Here's the drawing with two shaded views (mm, measured from the low corner). I have some questions. Coordinates: 2 decimals unless noted, no trailing zeros. Write each loop counter-clockwise with the first axis right and the second up, starting at its lowest first coordinate (ties: lowest second). Pieces come first, ordered by that corner, then holes. Notation, with made-up numbers: (78.25, -22) -> (85.25, -22) arc R18 cw to (85.25, 7) -> close; hole circle Ø6 at (-23, 7.25). An arc over 180 degrees is marked (long way). Put each result on its own line as item: value.
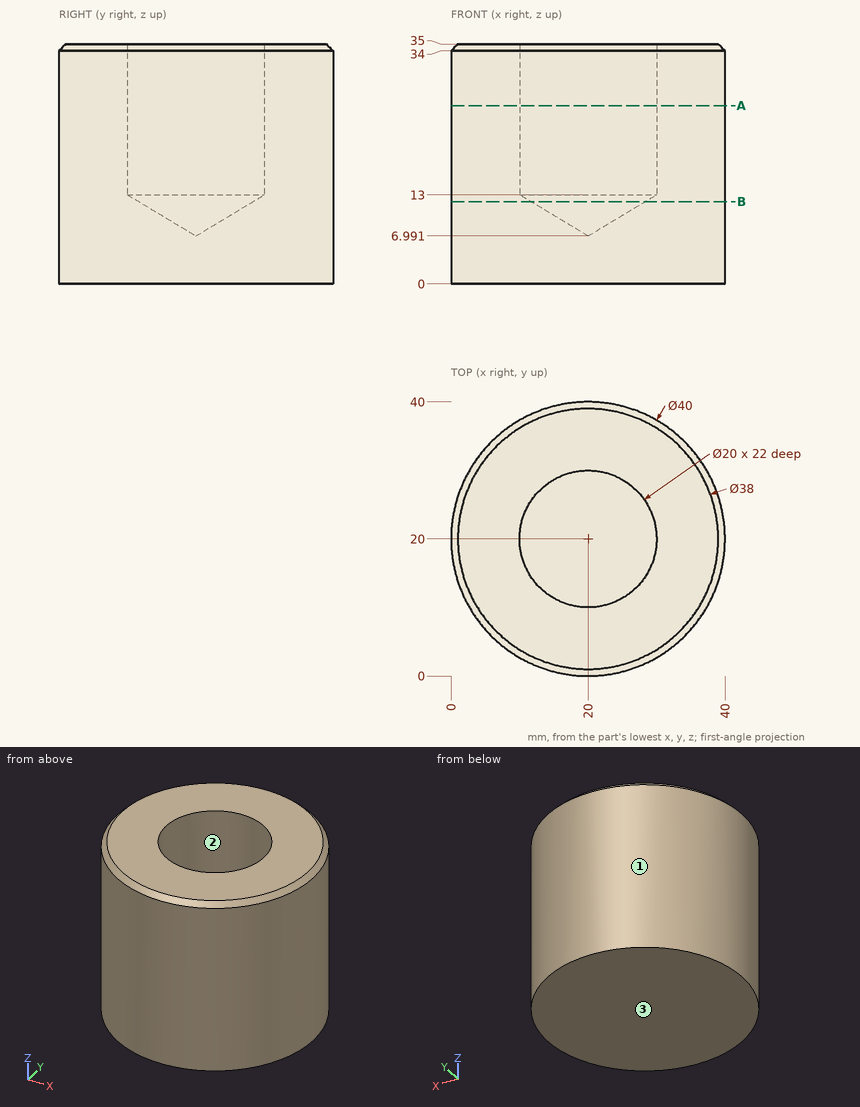
Item 1: Imagine slicing it at B-B on z = 12. Write out the boundary of the cut face in (x, y) (1 decimal).
Output:
outline: circle Ø40 at (20, 20); hole circle Ø16.7 at (20, 20)
Item 2: Please list where these lines run through material, in increasing order: line 1 along X through (y, z) = (20.5, 14); line 2 along Y through (x, z) = (20, 27); line 3 along X through (y, z) = (27, 29) (1 decimal). Write a range as from..to.
Output:
line 1: x = 0.01..10.01, 29.99..39.99
line 2: y = 0..10, 30..40
line 3: x = 1.3..12.9, 27.1..38.7
Item 3: Imagine slicing it at A-A on z = 26. Write out the boundary of the cut face in (x, y).
Output:
outline: circle Ø40 at (20, 20); hole circle Ø20 at (20, 20)
Item 4: For P1, Ø4, axis at x = 10.5, z = 24, coming from the -Y side; P2, Ø8, axis at x = 12, z = 18, coming from the -Y side; P3, Ø10, axis at x = 32, z = 5, coming from the +Y side (1 decimal), each with a flat end and sliding along its axis, tell me the tip position at first contact or that it passes through.
Output:
P1: stops at y = 1.46
P2: stops at y = 0.4
P3: stops at y = 38.7
Item 5: If we mould it in two halves opening along X, with no side actions, what happens to the marked faces 1, 2 and 3? For each: released by +X, released by -X, zero draft, split by the parting line, or undercut.
Output:
face 1: split by the parting line
face 2: undercut
face 3: zero draft
